```python
from build123d import *

# Parameters (mm, degrees)
F0_W     = 7
F0_H     = 5
F0_H_2   = 10
F1_DEPTH = 3
F2_W     = 7
F2_H     = 5
F3_DEPTH = 20
F5_DEPTH = 5
F6_R     = 2
F7_DEPTH = 5
F8_R     = 2
F9_DEPTH = 3


with BuildPart() as f1:
    # F0 (on Top) → F1 (new body)
    with BuildSketch(Plane.XY):
        with Locations((-4.6964466444, 11.5613198653)):
            Rectangle(F0_W, F0_H)
        with Locations((-4.6964466444, 4.0613198653)):
            Rectangle(F0_W, F0_H_2)
    extrude(amount=F1_DEPTH)

    # F2 (on face) → F3 (join)
    with BuildSketch(Plane.XY.offset(3)):
        with Locations((-4.6964466444, 11.5613198653)):
            Rectangle(F2_W, F2_H)
    extrude(amount=F3_DEPTH)

    # F4 (on face) → F5 (join, through all)
    with BuildSketch(Plane(origin=(0, 14.0613198653, 0), x_dir=(-1, 0, 0), z_dir=(0, 1, 0))):
        with BuildLine():
            Line((1.1964466444, 23), (8.1964466444, 23))
            ThreePointArc((8.1964466444, 23), (4.6964466444, 26.5), (1.1964466444, 23))
        make_face()
    extrude(amount=-F5_DEPTH)

    # F6 (on face) → F7 (cut, through all)
    with BuildSketch(Plane(origin=(0, 14.0613198653, 0), x_dir=(-1, 0, 0), z_dir=(0, 1, 0))):
        with Locations((4.6964466444, 23)):
            Circle(F6_R)
    extrude(amount=-F7_DEPTH, mode=Mode.SUBTRACT)

    # F8 (on face) → F9 (cut, through all)
    with BuildSketch(Plane.XY.offset(3)):
        with Locations((-4.6964466444, 4.0613198653)):
            Circle(F8_R)
    extrude(amount=-F9_DEPTH, mode=Mode.SUBTRACT)


solid = f1.part
```
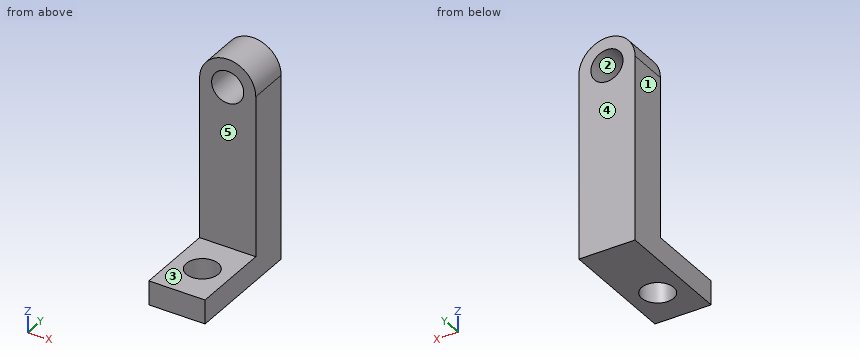
Design review of the part built by this model. Coordinates are the model's own, in mm. Face numbers are marked on the shaded views. A direction names the side the tool comes from. Coordinates: 2 decimals unless noted, no trailing zeros. Order: outer loops, then holes, each group sorted by start corner. A loop starts at its lowest first (then second) coordinate and runs counter-clockwise, first axis right, second up.
1) Mouldability with a two-part tool opening along Z and no side actions: class the marked faces 1, 2 and 3 as +Z half, -Z half, draft (parallel to the pull), parting line (faces both ways), or undercut.
2) Wall thickness on line 1 along Z through (x, y) = (-4.75, 12.25); line 2 along Z through (x, y) = (-7.5, 2); line 3 along Y through (x, z) = (-6, 19): over which ranges is each line inside the solid? List them lowest first.
3) For the marked faces 4 and 5, list the 3-axis set-ups (+Z, -Z, +X, -X, +Y, -Y) from which the entire face can be reached by the end or side of a thin tool; tool diameter is ignored.
4) Take a section at A-A, the plane y = 9.75. Give the boundary of the cut face in (x, z), and give its area (3 significant figures).
5) Take a section at B-B, the plane x = -5. Give the boundary of the cut face in (y, z), and give its area (3 significant figures).
6) Clearance check with flat-ended pins moving along their axes: pin 1 (2 mm diameter, centred on x = -6.5, y = 3.5, fed in from +Z); pin 2 (3 mm diameter, centred on x = -2.5, z = 17.5, fed in from -Y). State where each tip first meets the part, or that it passes through.
7) Take a section at C-C, the plane y = 3. Give the boundary of the cut face in (x, z), and give its area (3 significant figures).
8) Take a section at D-D, the plane z = 10.75. Give the boundary of the cut face in (x, y).
Returned:
1. face 1: draft
1. face 2: undercut
1. face 3: +Z half
2. line 1: z = 0 to 21, 25 to 26.5
2. line 2: z = 0 to 3
2. line 3: y = 9.06 to 14.06
3. face 4: +Z, -Z, +X, -X, +Y
3. face 5: +Z, +X, -X, -Y
4. outline: (-8.2, 0) - (-1.2, 0) - (-1.2, 23) arc R3.5 ccw to (-8.2, 23) - close; hole circle Ø4 at (-4.7, 23)
4. area: 168 mm2
5. outline: (-0.94, 0) - (2.08, 0) - (2.08, 3) - (-0.94, 3) - close; (6.04, 0) - (14.06, 0) - (14.06, 21.02) - (9.06, 21.02) - (9.06, 3) - (6.04, 3) - close; (9.06, 24.98) - (14.06, 24.98) - (14.06, 26.49) - (9.06, 26.49) - close
5. area: 131 mm2
6. pin 1: stops at z = 3
6. pin 2: stops at y = 9.06
7. outline: (-8.2, 0) - (-6.39, 0) - (-6.39, 3) - (-8.2, 3) - close; (-3, 0) - (-1.2, 0) - (-1.2, 3) - (-3, 3) - close
7. area: 10.8 mm2
8. outline: (-8.2, 9.06) - (-1.2, 9.06) - (-1.2, 14.06) - (-8.2, 14.06) - close
